Can you work these out from the model? Positions are in its coordinate system, mm. Give positions to 0.01 mm unless a question says otherwise; leave off trailing zeros. Order: outer loops, then holes, each group sorted by start corner. A loop starts at its lowest first (then second) coordinate and runs counter-clockwise, first axis right, second up.
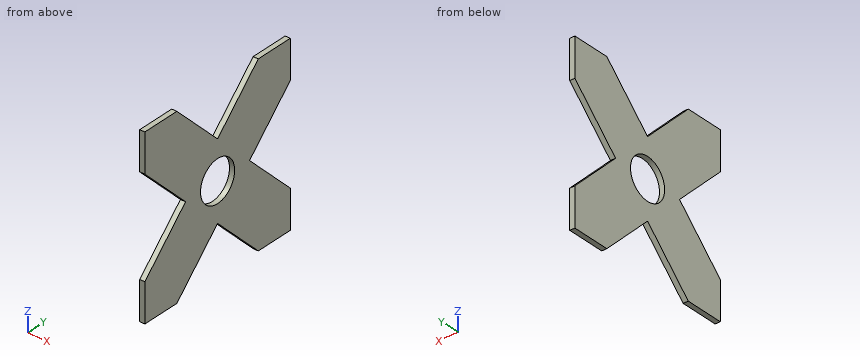
```python
from build123d import *

# Parameters (mm, degrees)
BOSS_EXTRUDE2_DEPTH = 10
SKETCH3_R           = 40
CUT_EXTRUDE1_DEPTH  = 10


with BuildPart() as part:
    # Sketch1 → Boss-Extrude2 (new body)
    with BuildSketch(Plane(origin=(0, 0, 0), x_dir=(0, 0, -1), z_dir=(1, 0, 0))):
        Polygon((0, 0), (75, 0), (170.45941546, 95.45941546), (265.91883092, 0), (340.91883092, 0), (340.91883092, 75), (245.45941546, 170.45941546), (340.91883092, 265.91883092), (340.91883092, 340.91883092), (265.91883092, 340.91883092), (170.45941546, 245.45941546), (75, 340.91883092), (0, 340.91883092), (0, 265.91883092), (95.45941546, 170.45941546), (0, 75), align=None)
    extrude(amount=BOSS_EXTRUDE2_DEPTH)

    # Sketch3 → Cut-Extrude1 (cut)
    with BuildSketch(Plane(origin=(10, 0, 0), x_dir=(0, 0, -1), z_dir=(1, 0, 0))):
        with Locations((170.45941546, 170.45941546)):
            Circle(SKETCH3_R)
    extrude(amount=-CUT_EXTRUDE1_DEPTH, mode=Mode.SUBTRACT)


solid = part.part
```
1) If I drill on line 1 (Y direction, x = 2.75, z = -78); line 2 (Z direction, x = 4.5, y = 316.5); line 3 (Y direction, x = 2.5, z = -285), over which ranges is the centre line in solid material (lowest first)?
2) I'm going to push flat-ended pins straight in: pin 1 Ø6 at (x, y) = (5, 261.5) entering from -Z; pin 2 Ø6 at (x, z) = (6, -166) entering from -Y; pin 3 Ø3 at (x, z) = (3, -249) entering from -Y. Where does each tip first touch, or does it pass through?
3) Suppose I cut it at C-C (z = -26.5). Please give me the cut outline in (x, y).
4) Suppose I cut it at A-A (x = 7.75). Please give me the cut outline in (y, z), and give its area (3 significant figures).
5) Suppose I cut it at B-B (y = 42). Please give me the cut outline in (x, z).
6) Suppose I cut it at D-D (y = 106.5). Please give me the cut outline in (x, z).
Results:
1. line 1: y = 3 to 153, 187.92 to 337.92
1. line 2: z = -340.92 to -241.5, -99.42 to 0
1. line 3: y = 0 to 130.92, 210 to 340.92
2. pin 1: stops at z = -339.5
2. pin 2: stops at y = 88
2. pin 3: stops at y = 15.42
3. outline: (0, 0) - (10, 0) - (10, 101.5) - (0, 101.5) - close; (0, 239.42) - (10, 239.42) - (10, 340.92) - (0, 340.92) - close
4. outline: (0, -340.92) - (75, -340.92) - (170.46, -245.46) - (265.92, -340.92) - (340.92, -340.92) - (340.92, -265.92) - (245.46, -170.46) - (340.92, -75) - (340.92, 0) - (265.92, 0) - (170.46, -95.46) - (75, 0) - (0, 0) - (0, -75) - (95.46, -170.46) - (0, -265.92) - close; hole circle Ø80 at (170.46, -170.46)
4. area: 74,700 mm2
5. outline: (0, -340.92) - (10, -340.92) - (10, -223.92) - (0, -223.92) - close; (0, -117) - (10, -117) - (10, 0) - (0, 0) - close
6. outline: (0, -309.42) - (10, -309.42) - (10, -31.5) - (0, -31.5) - close
